from build123d import *

# Parameters (mm, degrees)
F0_W     = 89
F0_H     = 75
F1_DEPTH = 4.8
F2_W     = 75
F2_H     = 1.4
F3_DEPTH = 2
F4_R     = 1.99999


# Not quite as in the source:
# - a fillet or chamfer is up to 0.001 mm smaller than in the source, because OpenCascade refuses the exact size


with BuildPart() as f1:
    # F0 (on Front) → F1 (new body)
    with BuildSketch(Plane.XZ):
        Rectangle(F0_W, F0_H)
    extrude(amount=F1_DEPTH)

    # F2 (on face) → F3 (cut)
    with BuildSketch(Plane.XZ.offset(4.8)):
        Polygon((-42.5, 37.5), (-42.5, -37.5), (-37.5, -37.5), (-37.5, 12.5), (-37.5, 13.9), (-37.5, 37.5), align=None)
        with Locations((0, 13.2)):
            Rectangle(F2_W, F2_H)
        Polygon((37.5, 13.9), (37.5, 12.5), (37.5, -37.5), (42.5, -37.5), (42.5, 37.5), (37.5, 37.5), align=None)
    extrude(amount=-F3_DEPTH, mode=Mode.SUBTRACT)

    # F4 (radius 2 in the source; OpenCascade refuses exactly that, so slightly less here)
    f4_edges = [f1.edges().sort_by_distance(p)[0] for p in [
        (-44.5, -4.8, 0),
        (44.5, -4.8, 0),
        (44.5, 0, 0),
        (-44.5, 0, 0),
    ]]
    fillet(f4_edges, radius=F4_R)


solid = f1.part
Could you check a few things on this model? Use its own coordinates, in mm. A direction names the side the tool comes from. Give positions to 0.01 mm unless a question says otherwise; leave off trailing zeros. Order: outer loops, then holes, each group sorted by start corner. A loop starts at its lowest first (then second) coordinate and runs counter-clockwise, first axis right, second up. Notation, with made-up numbers: (86, -2.5) - (143, -2.5) arc R35 cw to (143, 34.5) - close; hole circle Ø4 at (3, 12.25). An arc over 180 degrees is marked (long way). Return JSON: item names as keys, results as strings. Group by question number.
Q1. Suppose I cut it at A-A, the plane y = -3.8. Please give me the cut outline in (x, z), and give its area (3 significant figures).
Q2. Thinking about a two-plate mould opening in Z: for faces 3 (the face through (-1, -2, 37.5)), 4 (the face through (-43.93, -4.2, 0.52)), 5 (the face through (-1, -4, 12.5)), 6 (the face through (-1, -4, 13.9)), which applies, pulls with the +Z half, pulls with the -Z half, needs draft (parallel to the pull), parting line crosses it, or undercut?
Q3. Will these pins go through, and if not, where does the flat tip stop? pin 1 Ø2 at (y, z) = (-4, 27.5) entering from +X; pin 2 Ø1 at (y, z) = (-4, 18.5) entering from -X; pin 3 Ø1 at (y, z) = (-4, 3) entering from +X.
Q4. Which directions (+Z, -Z, +X, -X, +Y, -Y) give clear straight access to the entire face, cutting with the end or side of a thin tool? Please do faces 1 (the face through (-1, -2, -37.5)), 2 (the face through (37.5, -4, 26)).
Q5. Please list where these lines run through material, in increasing order: line 1 along Z through (x, y) = (-35.5, -4.25); line 2 along X through (y, z) = (-4.55, -20); line 3 along X through (y, z) = (-3.9, 4). Write a range as [from, to].
Resolved:
{
 "1": {"outline": "(-44.23, -37.5) - (-42.5, -37.5) - (-42.5, 37.5) - (-44.23, 37.5) - close; (-37.5, -37.5) - (37.5, -37.5) - (37.5, 12.5) - (-37.5, 12.5) - close; (-37.5, 13.9) - (37.5, 13.9) - (37.5, 37.5) - (-37.5, 37.5) - close; (42.5, -37.5) - (44.23, -37.5) - (44.23, 37.5) - (42.5, 37.5) - close", "area": "5,780 mm2"},
 "2": {"face 3": "pulls with the +Z half", "face 4": "needs draft", "face 5": "undercut", "face 6": "undercut"},
 "3": {"pin 1": "stops at x = 44.49", "pin 2": "stops at x = -44.37", "pin 3": "stops at x = 44.37"},
 "4": {"face 1": "-Z, +X, -X, +Y, -Y", "face 2": "+Z, -Z, -Y"},
 "5": {"line 1": "z = [-37.5, 12.5], [13.9, 37.5]", "line 2": "x = [-43.47, -42.5], [-37.5, 37.5], [42.5, 43.47]", "line 3": "x = [-44.17, -42.5], [-37.5, 37.5], [42.5, 44.17]"}
}
